Design review of the part built by this model. Coordinates are the model's own, in mm. A direction names the side the tool comes from. Coordinates: 2 decimals unless noted, no trailing zeros. Loops run counter-clockwise (first coordinate to the right, second up) from the corner with the lowest first, then second, coordinate; pieces in that order, holes last. Notation, with made-up numbers: (-38, 30) -> (-33, 30) arc R19 cw to (-33, 37) -> close; hole circle Ø11 at (-16, -11). An arc over 180 degrees is marked (long way). One line per item, written item: value. Start each with the question number.
1. For probe 1 along X at (y, z) = (19, 1.8); probe 2 along Y at (x, z) = (10, 0.6); probe 3 along X at (y, z) = (-14, 0.55), list the stretches that pass through material, from the lowest coordinate up.
2. Add section D-D on x = 2. Write out the cut boundary in (y, z), plus the area to 3 significant figures.
3. Insertion check: pin 1 (8 mm diameter, centred on x = 22.5, y = 19.5, fed in from +Z); pin 2 (2 mm diameter, centred on y = 10, z = 5, fed in from +X); pin 3 (5 mm diameter, centred on x = -27.5, y = -19.5, fed in from +Z). Each pin has a flat end and moves straight along its axis. Give the tip position at first contact, or say it passes through.
4. Add section C-C on z = 1.4. Write out the cut boundary in (x, y).
5. Add section A-A on x = -30. Write out the cut boundary in (y, z), plus the area to 3 significant figures.
6. Machinability: for faces 1 (the flat face through (-5, -28, 3)), 2 (the flat face through (-21.61, 18.25, 2.29)), 3 (the flat face through (-27, -15, 3.5)), which of the approach directions +Z, -Z, +X, -X, +Y, -Y give a long, thin tool a straight path to every point of the face, cutting with its end or side? Answer none if there is none.
7. Add section B-B on y = 19. Write out the cut boundary in (x, z).
8. Draft analysis for pull direction Y (two halves, no side actions). For faces 4 (the flat face through (26.87, -9.74, 2.96)), 5 (the flat face through (-20.455, -11.891, 4.768)), 6 (the flat face through (-5, 28, 2)), 7 (the cylindrical face through (-15, 0, 3)), state which applies: pulls with the +Y half, pulls with the -Y half, needs draft (parallel to the pull), parting line crosses it, or undercut.
```python
from build123d import *

# Parameters (mm, degrees)
F1_DEPTH = 6
F2_R     = 5
F4_DEPTH = 2.5
F5_DEPTH = 2
F3_W     = 10
F3_H     = 15
F6_DEPTH = 1.5
F7_DEPTH = 1
F8_DEPTH = 0.5


with BuildPart() as f1:
    # F0 (on Top) → F1 (new body)
    with BuildSketch(Plane.XY):
        Polygon((5, 38.660254), (-5, 38.660254), (-5, 8.660254), (-30.980762, 23.660254), (-35.980762, 15), (-10, 0), (-35.980762, -15), (-30.980762, -23.660254), (-5, -8.660254), (-5, -38.660254), (5, -38.660254), (5, -8.660254), (30.980762, -23.660254), (35.980762, -15), (10, 0), (35.980762, 15), (30.980762, 23.660254), (5, 8.660254), align=None)
    extrude(amount=F1_DEPTH)

    # F2
    f2_edges = [f1.edges().sort_by_distance(p)[0] for p in [
        (-5, 8.660254, 3),
        (5, 8.660254, 3),
        (10, 0, 3),
        (5, -8.660254, 3),
        (-5, -8.660254, 3),
        (-10, 0, 3),
    ]]
    fillet(f2_edges, radius=F2_R)

    # F3 (on face) → F4 (cut)
    with BuildSketch(Plane.XY.offset(6)):
        Polygon((-35.980762, -15), (-30.980762, -23.660254), (-17.990381, -16.160254), (-22.990381, -7.5), align=None)
    extrude(amount=-F4_DEPTH, mode=Mode.SUBTRACT)

    # F3 (on face) → F5 (cut)
    with BuildSketch(Plane.XY.offset(6)):
        Polygon((-35.980762, 15), (-22.990381, 7.5), (-17.990381, 16.160254), (-30.980762, 23.660254), align=None)
    extrude(amount=-F5_DEPTH, mode=Mode.SUBTRACT)

    # F3 (on face) → F6 (cut)
    with BuildSketch(Plane.XY.offset(6)):
        with Locations((0, 31.160254)):
            Rectangle(F3_W, F3_H)
    extrude(amount=-F6_DEPTH, mode=Mode.SUBTRACT)

    # F3 (on face) → F7 (cut)
    with BuildSketch(Plane.XY.offset(6)):
        Polygon((17.990381, 16.160254), (22.990381, 7.5), (35.980762, 15), (30.980762, 23.660254), align=None)
    extrude(amount=-F7_DEPTH, mode=Mode.SUBTRACT)

    # F3 (on face) → F8 (cut)
    with BuildSketch(Plane.XY.offset(6)):
        Polygon((22.990381, -7.5), (17.990381, -16.160254), (30.980762, -23.660254), (35.980762, -15), align=None)
    extrude(amount=-F8_DEPTH, mode=Mode.SUBTRACT)


solid = f1.part
```
Worked answers:
1. probe 1: x = -33.67 to -22.91, -5 to 5, 22.91 to 33.67
1. probe 2: y = -12.32 to 12.32
1. probe 3: x = -34.25 to -14.25, -6.26 to 6.26, 14.25 to 34.25
2. outline: (-38.66, 0) -> (38.66, 0) -> (38.66, 4.5) -> (23.66, 4.5) -> (23.66, 6) -> (-38.66, 6) -> close
2. area: 441 mm²
3. pin 1: stops at z = 5
3. pin 2: stops at x = 29.05
3. pin 3: stops at z = 3.5
4. outline: (-35.98, -15) -> (-30.98, -23.66) -> (-12.5, -12.99) arc R5 cw to (-5, -17.32) -> (-5, -38.66) -> (5, -38.66) -> (5, -17.32) arc R5 cw to (12.5, -12.99) -> (30.98, -23.66) -> (35.98, -15) -> (17.5, -4.33) arc R5 cw to (17.5, 4.33) -> (35.98, 15) -> (30.98, 23.66) -> (12.5, 12.99) arc R5 cw to (5, 17.32) -> (5, 38.66) -> (-5, 38.66) -> (-5, 17.32) arc R5 cw to (-12.5, 12.99) -> (-30.98, 23.66) -> (-35.98, 15) -> (-17.5, 4.33) arc R5 cw to (-17.5, -4.33) -> close
5. outline: (-23.09, 0) -> (-11.55, 0) -> (-11.55, 3.5) -> (-23.09, 3.5) -> close; (11.55, 0) -> (23.09, 0) -> (23.09, 4) -> (11.55, 4) -> close
5. area: 86.6 mm²
6. face 1: +Z, -Z, -Y
6. face 2: +Z, -Z, +Y
6. face 3: +Z, -X, -Y
7. outline: (-33.67, 0) -> (-22.91, 0) -> (-22.91, 4) -> (-33.67, 4) -> close; (-5, 0) -> (5, 0) -> (5, 6) -> (-5, 6) -> close; (22.91, 0) -> (33.67, 0) -> (33.67, 5) -> (22.91, 5) -> close
8. face 4: undercut
8. face 5: pulls with the -Y half
8. face 6: needs draft
8. face 7: undercut
